Build history of the part. All positions in model axes, mm. Face numbers are marked on the shaded views. Coordinates: 2 decimals unless noted, no trailing zeros. Order: outer loops, then holes, each group sorted by start corner. A loop starts at its lowest first (then second) coordinate and runs counter-clockwise, first axis right, second up. Notation, with made-up numbers: M 47,75.5 L 70,75.5 A19 ccw 70,79.5 Z; hole C 17.25,39.25 d10. An arc over 180 degrees is marked long. Write item = value, one per line. Start each with the question number.
Q1. Pin check, flat tips, straight feed: P1, Ø10, axis at y = -42.5, z = 32, coming from the -X side; P2, Ø10, axis at y = -62, z = 58, coming from the -X side; P3, Ø6, axis at x = -186, z = 43.5, coming from the -Y side; P4, Ø10, axis at x = 179, z = 3.5, coming from the +Y side. Stop position of each tip, or through.
Q2. Pull direction Z, two halves, no side cores. Call the marked faces 1, 2, 3 and 4: released by +Z, released by -Z, zero draft, split by the parting line, or undercut.
Q3. Drill centre lines: probe 1 along Z at (x, y) = (-117, -32.5); probe 2 along Y at (x, z) = (-103, -42.5); probe 3 along X at (y, z) = (-19, -33). Where is each one in solid material? Low to high.
Q4. Band-saw the part on A-A on x = -12. Write the cut outline in (y, z), plus the area to 3 significant figures.
```python
from build123d import *

# Parameters (mm, degrees)
F0_W     = 367.0583882955
F0_H     = 150
F1_DEPTH = 70
F1_TAPER = -40
F3_DEPTH = 180.4313063622
F4_T     = -2.54


with BuildPart() as f1:
    # F0 (on Front) → F1 (new body)
    with BuildSketch(Plane.XZ):
        Rectangle(F0_W, F0_H)
    extrude(amount=F1_DEPTH, taper=F1_TAPER)

    # F2 (on face) → F3 (cut)
    with BuildSketch(Plane(origin=(0, 0, 0), x_dir=(-1, 0, 0), z_dir=(0, 1, 0))):
        Polygon((273.2922434807, -75), (183.5291941477, -75), (-183.5291941477, -75), (-315.6023919582, -75), (-315.6023919582, -152.7352780104), (273.2922434807, -152.7352780104), align=None)
        Polygon((183.5291941477, 75), (257.0646107197, 75), (257.0646107197, 213.5136723518), (-302.473783493, 213.5136723518), (-302.473783493, 75), (-183.5291941477, 75), align=None)
    extrude(amount=-F3_DEPTH, mode=Mode.SUBTRACT)

    # F4
    f4_openings = [f1.faces().sort_by_distance(p)[0] for p in [
        (0, -70, 0),
    ]]
    offset(amount=F4_T, openings=f4_openings, kind=Kind.INTERSECTION)


solid = f1.part
```
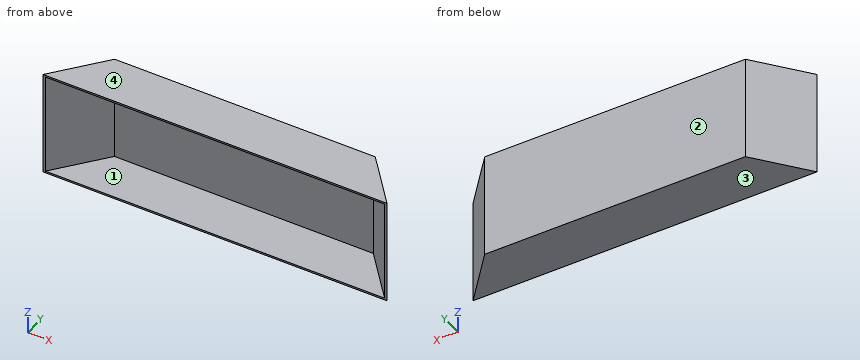
Recorded:
q1.P1 = -223.39
q1.P2 = -239.75
q1.P3 = -10.47
q1.P4 = 0
q2.face_1 = undercut
q2.face_2 = zero draft
q2.face_3 = released by -Z
q2.face_4 = released by +Z
q3.probe_1 = -75 to -72.46, 72.46 to 75
q3.probe_2 = -2.54 to 0
q3.probe_3 = -199.47 to -196.16, 196.16 to 199.47
q4.outline = M -70,-75 L 0,-75 L 0,75 L -70,75 L -70,72.46 L -2.54,72.46 L -2.54,-72.46 L -70,-72.46 Z
q4.area = 724 mm2
